from build123d import *

# Parameters (mm, degrees)
BOSS_EXTRUDE1_DEPTH = 20


with BuildPart() as part:
    # Sketch1 → Boss-Extrude1 (new body)
    with BuildSketch(Plane.XY):
        with BuildLine():
            Line((130.834806192, 133.228481614), (80.834806192, 133.228481614))
            Line((80.834806192, 133.228481614), (80.834806192, 105.140286594))
            Line((80.834806192, 105.140286594), (120.834806192, 105.140286594))
            Line((120.834806192, 105.140286594), (120.834806192, 74.834602493))
            Line((120.834806192, 74.834602493), (80.834806192, 74.834602493))
            Line((80.834806192, 74.834602493), (80.834806192, 68.182135251))
            Line((80.834806192, 68.182135251), (130.834806192, 68.182135251))
            Line((130.834806192, 68.182135251), (130.834806192, 105.488568969))
            ThreePointArc((130.834806192, 105.488568969), (127.905874004, 112.559636781), (120.834806192, 115.488568969))
            Line((120.834806192, 115.488568969), (90.074344028, 115.488568969))
            Line((90.074344028, 115.488568969), (90.074344028, 126.576014372))
            Line((90.074344028, 126.576014372), (130.834806192, 126.576014372))
            Line((130.834806192, 126.576014372), (130.834806192, 133.228481614))
        make_face()
    extrude(amount=BOSS_EXTRUDE1_DEPTH)


solid = part.part
Build history of the part. All positions in model axes, mm. A direction names the side the tool comes from. Coordinates: 2 decimals unless noted, no trailing zeros. Order: outer loops, then holes, each group sorted by start corner. A loop starts at its lowest first (then second) coordinate and runs counter-clockwise, first axis right, second up. Notation, with made-up numbers: (-25, -35) -> (7, -35) arc R21 cw to (7, -14) -> close; hole circle Ø4 at (55, 63). An arc over 180 degrees is marked (long way). One line per item, written item: value.
(1) Probe line 1 (Y direction, x = 110.5, z = 14.75); line 2 (X direction, y = 102, z = 16.5); line 3 (X direction, y = 119, z = 4.5). List the from-to ranges inside material, lowest first. Write a range as [from, to].
Checked values:
line 1: [68.18, 74.83], [105.14, 115.49], [126.58, 133.23]
line 2: [120.83, 130.83]
line 3: [80.83, 90.07]
(2) Mould opens along Y. For faces 4 (the flat face through (106, 133.228, 10)), 5 (the flat face through (80.835, 119, 10)), 6 (the flat face through (101, 105.14, 10)) say: pulls with the +Y half, pulls with the -Y half, needs draft (parallel to the pull), parting line crosses it, or undercut.
Checked values:
face 4: pulls with the +Y half
face 5: needs draft
face 6: undercut
(3) Slice it at B-B, the plane x = 89. List the corners of the cut face in (y, z).
Checked values:
outline: (68.18, 0) -> (74.83, 0) -> (74.83, 20) -> (68.18, 20) -> close; (105.14, 0) -> (133.23, 0) -> (133.23, 20) -> (105.14, 20) -> close
(4) Slice it at D-D, the plane x = 127. List the corners of the cut face in (y, z).
Checked values:
outline: (68.18, 0) -> (113.36, 0) -> (113.36, 20) -> (68.18, 20) -> close; (126.58, 0) -> (133.23, 0) -> (133.23, 20) -> (126.58, 20) -> close
(5) Tool access for faces 1 (the flat face through (101, 74.835, 10)), 2 (the flat face through (130.835, 87, 10)), 3 (the flat face through (90.074, 121, 10)): list every direction of +Z, -Z, +X, -X, +Y, -Y with a clear straight run to the whole face (end or side of a thin tool).
Checked values:
face 1: +Z, -Z, -X
face 2: +Z, -Z, +X, +Y, -Y
face 3: +Z, -Z, +X
(6) Slice it at A-A, the plane x = 115. List the corners of the cut face in (y, z), plus the area to 3 significant figures.
Checked values:
outline: (68.18, 0) -> (74.83, 0) -> (74.83, 20) -> (68.18, 20) -> close; (105.14, 0) -> (115.49, 0) -> (115.49, 20) -> (105.14, 20) -> close; (126.58, 0) -> (133.23, 0) -> (133.23, 20) -> (126.58, 20) -> close
area: 473 mm2
(7) Slice it at C-C, the plane z = 7. List the corners of the cut face in (x, y).
Checked values:
outline: (80.83, 68.18) -> (130.83, 68.18) -> (130.83, 105.49) arc R10 ccw to (120.83, 115.49) -> (90.07, 115.49) -> (90.07, 126.58) -> (130.83, 126.58) -> (130.83, 133.23) -> (80.83, 133.23) -> (80.83, 105.14) -> (120.83, 105.14) -> (120.83, 74.83) -> (80.83, 74.83) -> close
(8) Drop a flat-ended pin along its axis: pin 1 Ø12 at (y, z) = (122, 6) entering from +X. Give the stop position or say it passes through.
Checked values:
pin 1: x = 130.83
